Geometry: final body of the model. Coordinates: model frame, mm. Give positions to 0.01 mm unless a question says otherwise; leave off trailing zeros. Write each loop counter-clockwise with the first axis right and the second up, starting at its lowest first coordinate (ties: lowest second). Pieces come first, ordered by that corner, then holes.
Q1. Mould query, pull axis Y, two halves, no side actions, for faces 1 (the flat face through (-1, -22.5, 2)), 2 (the cylindrical face through (12.24, 19.483, 2.535)), 3 (the cylindrical face through (-43.76, 19.483, 2.535)), 4 (the flat face through (-1, 0, 0)). Classes: +Y half, -Y half, draft (parallel to the pull), parting line (faces both ways), or undercut.
Q2. Line query: line 1 (Y direction, x = -12.5, z = 3.85); line 2 (X direction, y = 19, z = 1.55); line 3 (Y direction, x = -13, z = 1.55). Output: solid intervals per line, ascending.
Q3. Section A-A (y = 17.5). Return the cut outline in (x, z), plus the area to 3 significant figures.
Q4. Section C-C (z = 3.05). State how many separate pieces and enclosed holes the cut face has, plus the area to 3 significant figures.
Q5. Pin query (flat end, axial travel): pin 1 Ø3 at (x, y) = (-12.5, 17.5) entering from -Z. Return the tip coordinate at first contact, or that it passes through.
Q6. Section B-B (x = 12.5). Return the cut outline in (y, z).
from build123d import *

# Parameters (mm, degrees)
SKETCH1_W           = 95
SKETCH1_H           = 45
BOSS_EXTRUDE1_DEPTH = 5
SKETCH2_R           = 2
CUT_EXTRUDE1_DEPTH  = 6


with BuildPart() as part:
    # Sketch1 → Boss-Extrude1 (new body)
    with BuildSketch(Plane.XY):
        Rectangle(SKETCH1_W, SKETCH1_H)
    extrude(amount=BOSS_EXTRUDE1_DEPTH)

    # Sketch2 → Cut-Extrude1 (cut, through all)
    with BuildSketch(Plane.XY.offset(5)):
        with Locations((43.5, 17.5)):
            Circle(SKETCH2_R)
        with Locations((43.5, -17.5)):
            Circle(SKETCH2_R)
        with Locations((12.5, -17.5)):
            Circle(SKETCH2_R)
        with Locations((12.5, 17.5)):
            Circle(SKETCH2_R)
        with Locations((-12.5, 17.5)):
            Circle(SKETCH2_R)
        with Locations((-12.5, -17.5)):
            Circle(SKETCH2_R)
        with Locations((-43.5, -17.5)):
            Circle(SKETCH2_R)
        with Locations((-43.5, 17.5)):
            Circle(SKETCH2_R)
    extrude(amount=-CUT_EXTRUDE1_DEPTH, mode=Mode.SUBTRACT)


solid = part.part
Computed:
1. face 1: -Y half
1. face 2: undercut
1. face 3: undercut
1. face 4: draft
2. line 1: y = -22.5 to -19.5, -15.5 to 15.5, 19.5 to 22.5
2. line 2: x = -47.5 to -44.82, -42.18 to -13.82, -11.18 to 11.18, 13.82 to 42.18, 44.82 to 47.5
2. line 3: y = -22.5 to -19.44, -15.56 to 15.56, 19.44 to 22.5
3. outline: (-47.5, 0) - (-45.5, 0) - (-45.5, 5) - (-47.5, 5) - close; (-41.5, 0) - (-14.5, 0) - (-14.5, 5) - (-41.5, 5) - close; (-10.5, 0) - (10.5, 0) - (10.5, 5) - (-10.5, 5) - close; (14.5, 0) - (41.5, 0) - (41.5, 5) - (14.5, 5) - close; (45.5, 0) - (47.5, 0) - (47.5, 5) - (45.5, 5) - close
3. area: 395 mm2
4. separate pieces: 1
4. enclosed holes: 8
4. area: 4,170 mm2
5. pin 1: passes through
6. outline: (-22.5, 0) - (-19.5, 0) - (-19.5, 5) - (-22.5, 5) - close; (-15.5, 0) - (15.5, 0) - (15.5, 5) - (-15.5, 5) - close; (19.5, 0) - (22.5, 0) - (22.5, 5) - (19.5, 5) - close
